Work out the finished part from the listing and answer in its coordinate system (mm). Face numbers are marked on the shaded views. Coordinates: 2 decimals unless noted, no trailing zeros. Loops run counter-clockwise (first coordinate to the right, second up) from the corner with the lowest first, then second, coordinate; pieces in that order, holes last. Notation, with made-up numbers: (38.25, 57.5) -> (80.25, 57.5) arc R13 ccw to (80.25, 64.5) -> close; hole circle Ø5 at (-13.5, 33.5). An arc over 180 degrees is marked (long way). Answer as CSV lines item,"result".
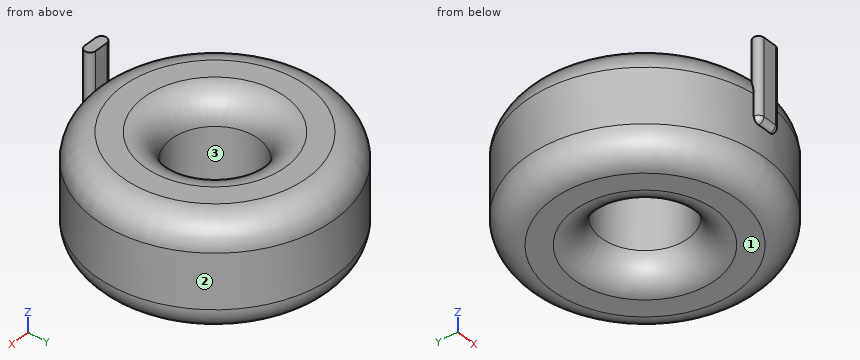
```python
from build123d import *

# Parameters (mm, degrees)
F0_R     = 44
F0_R_2   = 16
F1_DEPTH = 20
F2_R     = 10
F4_DEPTH = 30
F5_R     = 1.9999


# Not quite as in the source:
# - a fillet or chamfer is up to 0.001 mm smaller than in the source, because OpenCascade refuses the exact size


with BuildPart() as f1:
    # F0 (on Top) → F1 (new body, symmetric)
    with BuildSketch(Plane.XY):
        Circle(F0_R)
        Circle(F0_R_2, mode=Mode.SUBTRACT)
    extrude(amount=F1_DEPTH, both=True)

    # F2
    f2_edges = [f1.edges().sort_by_distance(p)[0] for p in [
        (-16, 0, 20),
        (16, 0, 0),
        (-16, 0, -20),
        (-44, 0, -20),
        (44, 0, 0),
        (-44, 0, 20),
    ]]
    fillet(f2_edges, radius=F2_R)

    # F3 (on Top) → F4 (join)
    with BuildSketch(Plane.XY):
        with BuildLine():
            Line((2.5, -41.9289198592), (-2.5, -41.9289198592))
            ThreePointArc((-2.5, -41.9289198592), (-4.5, -43.9289198592), (-2.5, -45.9289198592))
            Line((-2.5, -45.9289198592), (2.5, -45.9289198592))
            ThreePointArc((2.5, -45.9289198592), (4.5, -43.9289198592), (2.5, -41.9289198592))
        make_face()
    extrude(amount=F4_DEPTH)

    # F5 (radius 2 in the source; OpenCascade refuses exactly that, so slightly less here)
    f5_edges = [f1.edges().sort_by_distance(p)[0] for p in [
        (0, -45.92892, 0),
    ]]
    fillet(f5_edges, radius=F5_R)


solid = f1.part
```
(1) A cutting plane is placed at A-A, the plane y = 0. Write down the section's boundary in (x, z), and give its area (3 significant figures).
Computed values:
outline,"(-44, -10) arc R10 ccw to (-34, -20) -> (-26, -20) arc R10 ccw to (-16, -10) -> (-16, 10) arc R10 ccw to (-26, 20) -> (-34, 20) arc R10 ccw to (-44, 10) -> close; (16, -10) arc R10 ccw to (26, -20) -> (34, -20) arc R10 ccw to (44, -10) -> (44, 10) arc R10 ccw to (34, 20) -> (26, 20) arc R10 ccw to (16, 10) -> close"
area,"2,070 mm2"
(2) A cutting plane is placed at B-B, the plane z = -8. Write down the section's boundary in (x, y).
Computed values:
outline,"circle Ø88 at (0, 0); hole circle Ø32 at (0, 0)"
(3) For a pull along Y with two mould halves and no side action, classify the marked faces 1, 2 and 3 as pulls with the +Y half, pulls with the -Y half, needs draft (parallel to the pull), parting line crosses it, or undercut.
Computed values:
face 1,"needs draft"
face 2,"parting line crosses it"
face 3,"undercut"
(4) Consider line 1 along Y through (x, z) = (0, 4); line 2 along X through (y, z) = (-5.5, 9); line 3 along Y through (x, z) = (0, 0.5). Determine where each line is inside the solid, lowest interval first.
Computed values:
line 1,"-45.93 to -16, 16 to 44"
line 2,"-43.65 to -15.02, 15.02 to 43.65"
line 3,"-45.25 to -16, 16 to 44"
(5) A cutting plane is placed at D-D, the plane z = 7. Write down the section's boundary in (x, y).
Computed values:
outline,"(-4.49, -43.77) arc R2 ccw to (-2.5, -45.93) -> (2.5, -45.93) arc R2 ccw to (4.49, -43.77) arc R44 ccw (long way) to start; hole circle Ø32 at (0, 0)"
(6) Flat-ended cylindrical pins translate along their axes: pin 1 Ø8 at (y, z) = (3, -2) entering from +X; pin 2 Ø10 at (x, y) = (1.5, 18.5) entering from +Z; pin 3 Ø4 at (y, z) = (-28, 4) entering from +X; pin 4 Ø12 at (x, z) = (-19, 1.5) entering from -Y. Find the tip coordinate at first contact, or state that the pin passes through.
Computed values:
pin 1,"x = 44"
pin 2,"z = 19.7"
pin 3,"x = 35.5"
pin 4,"y = -42.04"
(7) A cutting plane is placed at C-C, the plane z = 25. Write down the section's boundary in (x, y).
Computed values:
outline,"(-2.5, -45.93) -> (2.5, -45.93) arc R2 ccw to (2.5, -41.93) -> (-2.5, -41.93) arc R2 ccw to start"
